For this review, take the finished solid that the model builds, in its own axes (mm). A direction names the side the tool comes from. Round coordinates to 2 decimals unless told otherwise and drop trailing zeros. Order: outer loops, then holes, each group sorted by start corner. A loop starts at its lowest first (then second) coordinate and runs counter-clockwise, first axis right, second up. Notation, with made-up numbers: M 79.25,39.25 L 135.25,39.25 A20 cw 135.25,65.25 Z; hole C 41.5,89.5 d11. An arc over 180 degrees is marked long. Answer as a JSON object with one key per item and string values.
from build123d import *

# Parameters (mm, degrees)
F1_DEPTH = 195
F2_R     = 3
F3_DEPTH = 25
F4_R     = 5
F5_DEPTH = 25


with BuildPart() as f1:
    # F0 (on Front) → F1 (new body)
    with BuildSketch(Plane.XZ):
        with BuildLine():
            Line((-1.160396, -84.100497), (-1.160396, 80.899503))
            Line((-1.160396, 80.899503), (-166.160396, 80.899503))
            Line((-166.160396, 80.899503), (-166.160396, 67.899503))
            Line((-166.160396, 67.899503), (-24.160396, 67.899503))
            ThreePointArc((-24.160396, 67.899503), (-17.089328, 64.970571), (-14.160396, 57.899503))
            Line((-14.160396, 57.899503), (-14.160396, -84.100497))
            Line((-14.160396, -84.100497), (-1.160396, -84.100497))
        make_face()
    extrude(amount=F1_DEPTH)

    # F2 (on face) → F3 (cut)
    with BuildSketch(Plane.XY.offset(80.899503)):
        with BuildLine():
            ThreePointArc((-150.911415, -25.154715), (-145.69743, -25.063704), (-140.483445, -25.154715))
            ThreePointArc((-140.483445, -25.154715), (-137.380574, -22.261241), (-140.274048, -19.15837))
            ThreePointArc((-140.274048, -19.15837), (-145.69743, -19.063704), (-151.120812, -19.15837))
            ThreePointArc((-151.120812, -19.15837), (-154.014286, -22.261241), (-150.911415, -25.154715))
        make_face()
        with BuildLine():
            ThreePointArc((-38.707305, -23.19722), (-44.051604, -19.555466), (-49.519744, -16.102444))
            ThreePointArc((-49.519744, -16.102444), (-53.641179, -17.109306), (-52.634317, -21.230741))
            ThreePointArc((-52.634317, -21.230741), (-47.343255, -24.571942), (-42.172023, -28.095764))
            ThreePointArc((-42.172023, -28.095764), (-37.990392, -27.378851), (-38.707305, -23.19722))
        make_face()
        with Locations((-145.69743, -174.463704)):
            Circle(F2_R)
    extrude(amount=-F3_DEPTH, mode=Mode.SUBTRACT)

    # F4 (on face) → F5 (cut)
    with BuildSketch(Plane.YZ.offset(-1.160396)):
        with Locations((-43.040507, 0)):
            Circle(F4_R)
    extrude(amount=-F5_DEPTH, mode=Mode.SUBTRACT)


solid = f1.part
1) Insertion check: P1, Ø12, axis at x = -54.5, y = -86.5, coming from the -Z side; P2, Ø3.5, axis at x = -145.7, y = -174.46, coming from the +Z side; P3, Ø8, axis at y = -87, z = 22.5, coming from the -X side. Each pin has a flat end and moves straight along its axis. Give the tip position at first contact, or say it passes through.
Geometry check:
{"P1": "stops at z = 67.9", "P2": "passes through", "P3": "stops at x = -14.16"}
2) Add section D-D on x = -18. State the section outline as (y, z) points, and give its area (3 significant figures).
Geometry check:
{"outline": "M -195,65.78 L 0,65.78 L 0,80.9 L -195,80.9 Z", "area": "2,950 mm²"}
3) Machinability: for faces 4 (the flat face through (-1.16, -96, -3)), 5 (the cylindrical face through (-43.976, -19.605, 74.491)), 6 (the flat face through (-14.16, -96, -12)), which of the approach directions +Z, -Z, +X, -X, +Y, -Y give a long, thin tool a straight path to every point of the face, cutting with its end or side? Answer none if there is none.
Geometry check:
{"face 4": "+Z, -Z, +X, +Y, -Y", "face 5": "+Z, -Z", "face 6": "-Z, -X, +Y, -Y"}
4) Add section C-C on x = -97.5. State the section outline as (y, z) points.
Geometry check:
{"outline": "M -195,67.9 L 0,67.9 L 0,80.9 L -195,80.9 Z"}
5) For L1, parallel to X at y = -91, z = -46.5; L2, parallel to Z at x = -80, y = -51, list the stretches that pass through material, from the lowest coordinate up.
Geometry check:
{"L1": "x = -14.16 to -1.16", "L2": "z = 67.9 to 80.9"}
6) Add section B-B on y = -67. State the section outline as (x, z) points, and give its area (3 significant figures).
Geometry check:
{"outline": "M -166.16,67.9 L -24.16,67.9 A10 cw -14.16,57.9 L -14.16,-84.1 L -1.16,-84.1 L -1.16,80.9 L -166.16,80.9 Z", "area": "4,140 mm²"}
7) Mouldability with a two-part tool opening along Y and no side actions: class faces 1 (the flat face through (-8, -96, -84.1)), 2 (the flat face through (-47, 0, 72)), 3 (the cylindrical face through (-148.695, -174.332, 74.491)) as +Y half, -Y half, draft (parallel to the pull), parting line (faces both ways), or undercut.
Geometry check:
{"face 1": "draft", "face 2": "+Y half", "face 3": "undercut"}
8) Add section A-A on z = 0. State the section outline as (x, y) points, and give its area (4 significant figures).
Geometry check:
{"outline": "M -14.16,-195 L -1.16,-195 L -1.16,-48.04 L -14.16,-48.04 Z; M -14.16,-38.04 L -1.16,-38.04 L -1.16,0 L -14.16,0 Z", "area": "2,405 mm²"}
